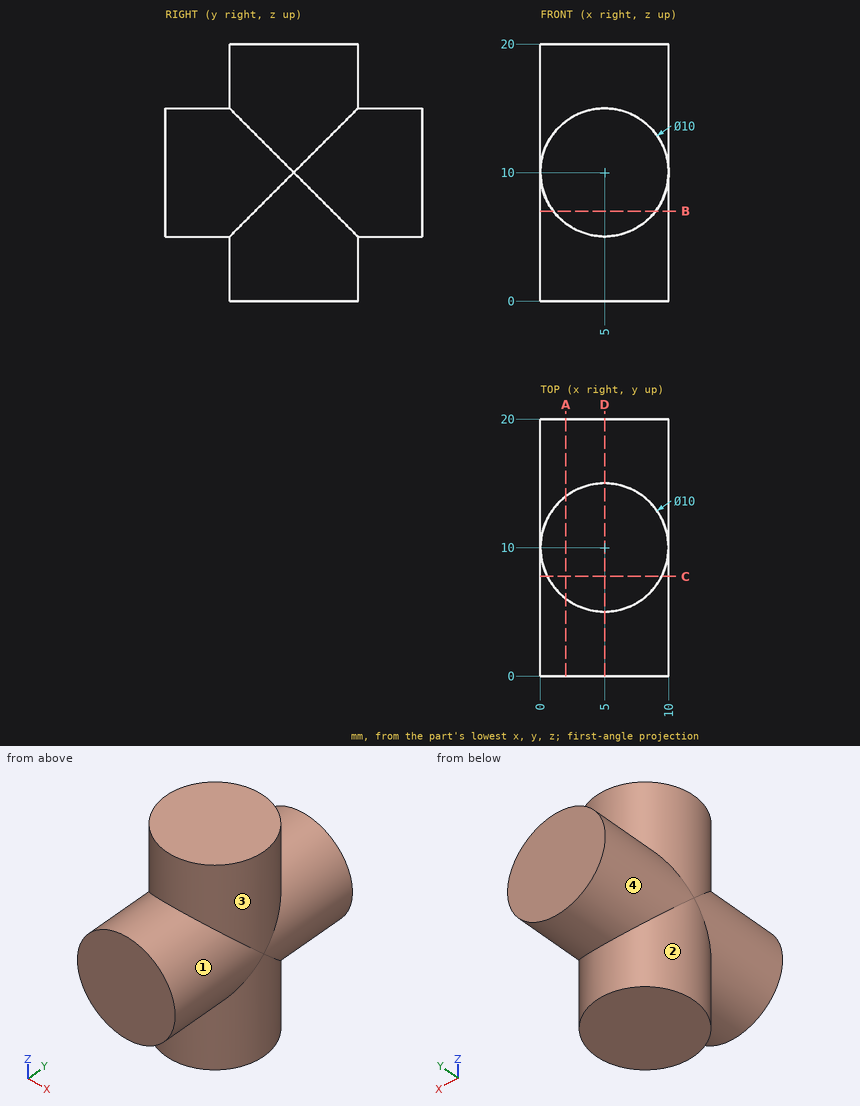
Input: dimensioned drawing with shaded views. Units: mm. Origin: part minimum x, y, z. A direction names the side the tool comes from. Give positions to 0.01 mm unless a question says otherwise; leave off trailing zeros. Loops run counter-clockwise (first coordinate to the right, second up) from the corner with the lowest first, then second, coordinate; pieces in that order, holes last. Notation, with made-up numbers: (70, 86.5) - (83, 86.5) arc R15 ccw to (83, 98.5) - close; hole circle Ø10 at (82, -36.5). An arc over 180 degrees is marked (long way). Answer as CSV lines item,"result". Start each with the question number.
(1) Ray query, line 1 along Z through (x, y) = (8, 16.25); line 2 along X through (y, z) = (1.5, 13.25); line 3 along Z through (x, y) = (1, 18.25). Return the intervals inside material, ascending. Write a range as [from, to].
(2) Section query D-D (x = 5). Output: boundary loops of the cut face in (y, z), and give its area (3 significant figures).
(3) Reachability of the marked faces 1, 2, 3 and 4 from +Z, -Z, +X, -X, +Y, -Y: full face, straight path, thin tool, end or side. Return the list, or none.
(4) Section query C-C (y = 7.75). Output: boundary loops of the cut face in (x, z), and give its area (3 significant figures).
(5) Section query A-A (x = 2). Output: boundary loops of the cut face in (y, z).
(6) Section query B-B (z = 7). Output: boundary loops of the cut face in (x, y).
(7) Pin query (flat end, axial travel): P1, Ø4, axis at y = 5, z = 2.5, coming from the +X side. Return the tip coordinate at first contact, or that it passes through.
Worked answers:
1,line 1,"z = [6, 14]"
1,line 2,"x = [1.2, 8.8]"
1,line 3,"z = [7, 13]"
2,outline,"(0, 5) - (5, 5) - (5, 0) - (15, 0) - (15, 5) - (20, 5) - (20, 15) - (15, 15) - (15, 20) - (5, 20) - (5, 15) - (0, 15) - close"
2,area,"300 mm^2"
3,face 1,"-Y"
3,face 2,"-Z"
3,face 3,"+Z"
3,face 4,"+Y"
4,outline,"(0.53, 0) - (9.47, 0) - (9.47, 7.75) arc R5 ccw to (9.47, 12.25) - (9.47, 20) - (0.53, 20) - (0.53, 12.25) arc R5 ccw to (0.53, 7.75) - close"
4,area,"182 mm^2"
5,outline,"(0, 6) - (6, 6) - (6, 0) - (14, 0) - (14, 6) - (20, 6) - (20, 14) - (14, 14) - (14, 20) - (6, 20) - (6, 14) - (0, 14) - close"
6,outline,"(1, 0) - (9, 0) - (9, 7) arc R5 ccw to (9, 13) - (9, 20) - (1, 20) - (1, 13) arc R5 ccw to (1, 7) - close"
7,P1,"stops at x = 9"
